Study the drawing (mm; zero at the part's minimum x, y, z) and answer. A direction names the side the tool comes from. Coordinates: 2 decimals unless noted, no trailing zeros. Answer in a Markdown table with one row per item. Add a question column.
Item 1: Straight lines are drawn through the part: line 1 (Y direction, x = 38.1, z = 3.5) (1 decimal); line 2 (Y direction, x = 40, z = 7.5) (1 decimal); line 3 (Y direction, x = 10, z = 26) (1 decimal). For each, find the intervals that lie inside material, in ascending order. Write a range as from..to.
Item 2: Given pin 1 Ø4 at (x, y) = (38, 3) entering from +Z; pin 2 Ø8 at (x, z) = (20, 3.5) entering from -Y; pin 3 Ø3 at (y, z) = (19.05, 20.62) entering from +X; pin 4 Ø10 at (x, y) = (25.5, 20) entering from +Z (1 decimal), each flat-ended and moving along its own axis, determine where each tip first touches the part or whether it passes through.
Item 3: Section A-A on x = 6.35 is taken. Count the separate pieces of the cut face and the enclosed holes in it, then the cut area to 3 significant figures.
Item 4: For a pull along X with two mould halves and no side action, classify the marked faces 5, 6, 7 and 8 as +X half, -X half, draft (parallel to the pull), parting line (faces both ways), or undercut.
Item 5: Which of the six approach directions +Z, -Z, +X, -X, +Y, -Y give full straight-line access (tool end or side, diameter ignored) to the marked faces 1, 2, 3 and 4?
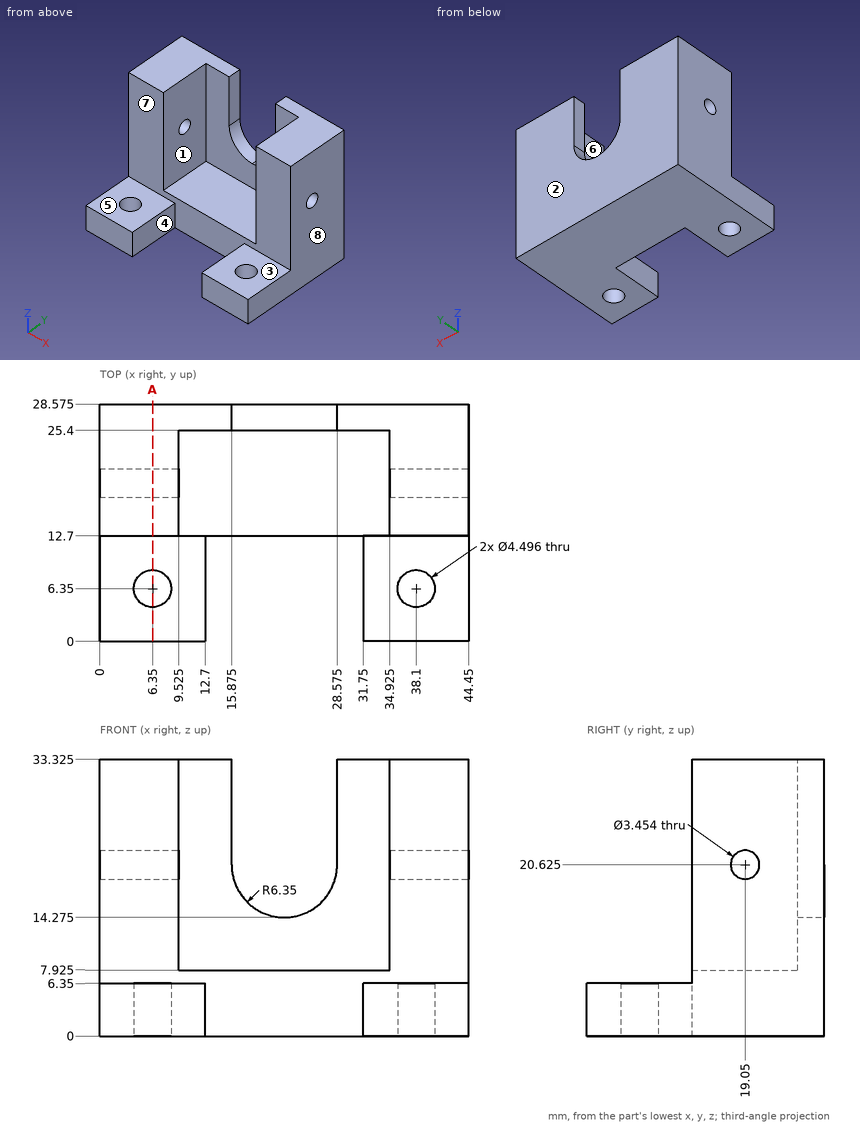
Results below:
| question | item | result |
|---|---|---|
| 1 | line 1 | y = 0..4.1, 8.6..28.6 |
| 1 | line 2 | y = 12.7..28.6 |
| 1 | line 3 | y = 25.4..28.6 |
| 2 | pin 1 | stops at z = 6.35 |
| 2 | pin 2 | stops at y = 12.7 |
| 2 | pin 3 | passes through |
| 2 | pin 4 | stops at z = 7.9 |
| 3 | separate pieces | 2 |
| 3 | enclosed holes | 1 |
| 3 | area | 572 mm2 |
| 4 | face 5 | draft |
| 4 | face 6 | undercut |
| 4 | face 7 | undercut |
| 4 | face 8 | +X half |
| 5 | face 1 | +Z, -Y |
| 5 | face 2 | +Z, -Z, +X, -X, +Y |
| 5 | face 3 | +Z, +X, -X, -Y |
| 5 | face 4 | +Z, -Z, -Y |
